from build123d import *

# Parameters (mm, degrees)
F1_DEPTH    = 63.5
F3_DEPTH    = 2.667
F5_T4_DEPTH = 71.247
F6_T4_DEPTH = 71.247
F8_D        = 6.35
F9_R        = 9.525


# Not quite as in the source:
# - a fillet or chamfer that OpenCascade refuses, or shapes differently, is made with other operations: its cross-section is extruded or revolved along the edge and cut away or added
# - a feature of the source that left no trace in its solid (it failed there, or was rolled back) is left out


with BuildPart() as f1:
    # F0 (on Front) → F1 (new body, symmetric)
    with BuildSketch(Plane.XZ):
        with BuildLine():
            Line((65.151, 0), (1.524, 0))
            ThreePointArc((1.524, 0), (0.4463692655, 0.4463692655), (0, 1.524))
            Line((0, 1.524), (0, 76.2))
            Line((0, 76.2), (0, 203.2))
            Line((0, 203.2), (-2.667, 203.2))
            Line((-2.667, 203.2), (-2.667, 76.2))
            Line((-2.667, 76.2), (-2.667, 1.524))
            ThreePointArc((-2.667, 1.524), (-1.43948452, -1.43948452), (1.524, -2.667))
            Line((1.524, -2.667), (65.151, -2.667))
            ThreePointArc((65.151, -2.667), (68.11448452, -1.43948452), (69.342, 1.524))
            Line((69.342, 1.524), (69.342, 76.2))
            Line((69.342, 76.2), (66.675, 76.2))
            Line((66.675, 76.2), (66.675, 1.524))
            ThreePointArc((66.675, 1.524), (66.2286307345, 0.4463692655), (65.151, 0))
        make_face()
    extrude(amount=F1_DEPTH, both=True)

    # F2 (on face) → F3 (join)
    with BuildSketch(Plane.XZ.offset(63.5)):
        with BuildLine():
            Line((66.6496, -1.143), (66.6496, 76.2))
            Line((66.6496, 76.2), (0.0254, 76.2))
            Line((0.0254, 76.2), (0.0254, -1.143))
            ThreePointArc((0.0254, -1.143), (0.4717692655, -2.2206307345), (1.5494, -2.667))
            Line((1.5494, -2.667), (65.1256, -2.667))
            ThreePointArc((65.1256, -2.667), (66.2032307345, -2.2206307345), (66.6496, -1.143))
        make_face()
    extrude(amount=-F3_DEPTH)

    # F4: F1 across plane


with BuildPart() as f1_1:
    add(f1.part)
    add(f1.part.mirror(Plane.XZ))

    # F5: fillet of radius 1.524 on 1 edges, made by hand


with BuildPart() as f5_tool2:
    # F5_s3 → F5_t4 (new body)
    with BuildSketch(Plane.YZ.offset(-2.286)):
        with BuildLine():
            ThreePointArc((-59.309, 0), (-60.3866307345, 0.4463692655), (-60.833, 1.524))
            Line((-60.833, 1.524), (-60.833, 0))
            Line((-60.833, 0), (-59.309, 0))
        make_face()
    extrude(amount=F5_T4_DEPTH)

    split(bisect_by=Plane.YZ.offset(0.0254), keep=Keep.TOP)

    split(bisect_by=Plane.YZ.offset(66.6496), keep=Keep.BOTTOM)


with BuildPart() as f1_2:
    add(f1_1.part)

    # F5_t1: union F5_tool2
    add(f5_tool2.part)

    # F6: fillet of radius 1.524 on 1 edges, made by hand


with BuildPart() as f6_tool2:
    # F6_s3 → F6_t4 (new body)
    with BuildSketch(Plane.YZ.offset(-2.286)):
        with BuildLine():
            ThreePointArc((59.309, 0), (60.3866307345, 0.4463692655), (60.833, 1.524))
            Line((60.833, 1.524), (60.833, 0))
            Line((60.833, 0), (59.309, 0))
        make_face()
    extrude(amount=F6_T4_DEPTH)

    split(bisect_by=Plane.YZ.offset(0.0254), keep=Keep.TOP)

    split(bisect_by=Plane.YZ.offset(66.6496), keep=Keep.BOTTOM)


with BuildPart() as f1_3:
    add(f1_2.part)

    # F6_t1: union F6_tool2
    add(f6_tool2.part)

    # F8 (through all)
    with Locations(Plane.YZ):
        with Locations((-44.45, 184.15), (44.45, 184.15)):
            Hole(F8_D / 2)

    # F9
    f9_edges = [f1_3.edges().sort_by_distance(p)[0] for p in [
        (-1.3335, -63.5, 203.2),
        (-1.3335, 63.5, 203.2),
    ]]
    fillet(f9_edges, radius=F9_R)


solid = f1_3.part
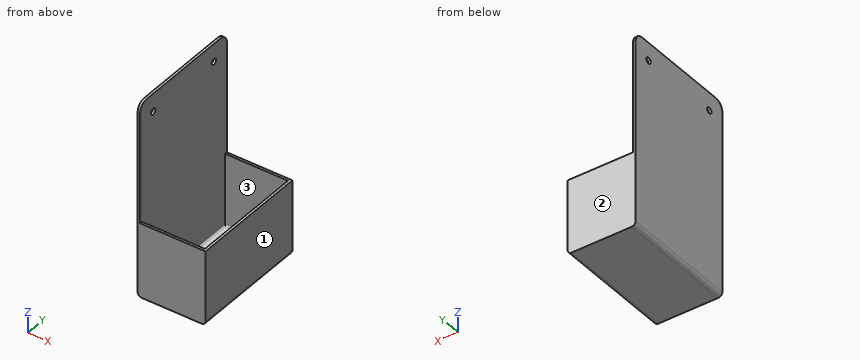
Can you work these out from the model? Positions are in its coordinate system, mm. Face numbers are marked on the shaded views. Give positions to 0.01 mm unless a question says otherwise; leave off trailing zeros. Order: outer loops, then holes, each group sorted by start corner. A loop starts at its lowest first (then second) coordinate and runs counter-clockwise, first axis right, second up. Notation, with made-up numbers: M 31,60.5 L 77,60.5 A25 ccw 77,74.5 Z; hole C 60,-17 d8. An arc over 180 degrees is marked long. Use a Markdown table: item, result. Add a question column.
Item 1: Will these pins go through, and if not, where does the flat tip stop? pin 1 (12 mm diameter, centred on y = -27, z = 145.5, fed in from +X); pin 2 (0.8 mm diameter, centred on x = 36.5, y = -62, fed in from +Z); pin 3 (8 mm diameter, centred on x = 46, y = -13, fed in from +Z).
Item 2: Suppose I cut it at D-D (x = 52). List the corners of the cut face in (y, z) for me, then the cut area to 3 significant figures.
Item 3: Suppose I cut it at B-B (y = 44.45). List the corners of the cut face in (x, z) for me (3 decimals).
Item 4: We'd pull the mould along X, two halves only. Please class the marked faces 1, 2 and 3: +X half, -X half, draft (parallel to the pull), parting line (faces both ways), or undercut.
Item 5: If I drill on L1, parallel to Y at x = -1, z = 184.15 (3 decimals); L2, parallel to Y at x = 61, z = 66; L3, parallel to X at y = 55, z = 17 (3 decimals), over which ranges is the centre line in solid material (lowest first)? Write a range as [from, to].
Item 6: Suppose I cut it at C-C (z = 184.15). List the corners of the cut face in (x, y) for me (3 decimals), then the cut area to 3 significant figures.
Item 7: Suppose I cut it at A-A (z = 68). List the corners of the cut face in (x, y) for me (3 decimals).
Answer sheet:
| question | item | result |
|---|---|---|
| 1 | pin 1 | stops at x = 0 |
| 1 | pin 2 | stops at z = 76.2 |
| 1 | pin 3 | stops at z = 0 |
| 2 | outline | M -63.5,-2.67 L 63.5,-2.67 L 63.5,76.2 L 60.83,76.2 L 60.83,1.52 A1.52 cw 59.31,0 L -59.31,0 A1.52 cw -60.83,1.52 L -60.83,76.2 L -63.5,76.2 Z |
| 2 | area | 746 mm² |
| 3 | outline | M -2.667,1.524 A4.191 ccw 1.524,-2.667 L 65.151,-2.667 A4.191 ccw 69.342,1.524 L 69.342,76.2 L 66.675,76.2 L 66.675,1.524 A1.524 cw 65.151,0 L 1.524,0 A1.524 cw 0,1.524 L 0,180.975 L -2.667,180.975 Z; M -2.667,187.325 L 0,187.325 L 0,203.2 L -2.667,203.2 Z |
| 4 | face 1 | +X half |
| 4 | face 2 | draft |
| 4 | face 3 | undercut |
| 5 | L1 | y = [-63.5, -47.625], [-41.275, 41.275], [47.625, 63.5] |
| 5 | L2 | y = [-63.5, -60.83], [60.83, 63.5] |
| 5 | L3 | x = [-2.667, 0], [66.675, 69.342] |
| 6 | outline | M -2.667,-63.5 L 0,-63.5 L 0,-47.625 L -2.667,-47.625 Z; M -2.667,-41.275 L 0,-41.275 L 0,41.275 L -2.667,41.275 Z; M -2.667,47.625 L 0,47.625 L 0,63.5 L -2.667,63.5 Z |
| 6 | area | 305 mm² |
| 7 | outline | M -2.667,-63.5 L 0,-63.5 L 0,63.5 L -2.667,63.5 Z; M 0.025,-63.5 L 66.65,-63.5 L 66.65,-60.833 L 0.025,-60.833 Z; M 0.025,60.833 L 66.65,60.833 L 66.65,63.5 L 0.025,63.5 Z; M 66.675,-63.5 L 69.342,-63.5 L 69.342,63.5 L 66.675,63.5 Z |
